Geometry: final body of the model. Coordinates: model frame, mm. A direction names the side the tool comes from. Round coordinates to 2 decimals unless told otherwise and drop trailing zeros. Write each loop counter-clockwise with the first axis right and the second up, starting at its lowest first coordinate (ties: lowest second). Pieces come first, ordered by that corner, then holes.
from build123d import *

# Parameters (mm, degrees)
SKETCH_R     = 3.65
PAD_DEPTH    = 31
SKETCH001_R  = 3.15
PAD001_DEPTH = 5
FILLET_R     = 1


with BuildPart() as part:
    # Sketch → Pad (new body)
    with BuildSketch(Plane.XY):
        Circle(SKETCH_R)
    extrude(amount=PAD_DEPTH)

    # Sketch001 (on Face3 of Pad) → Pad001 (join)
    with BuildSketch(Plane.XY.offset(31)):
        Circle(SKETCH001_R)
    extrude(amount=PAD001_DEPTH)

    # Fillet
    fillet_edges = [part.edges().sort_by_distance(p)[0] for p in [
        (-3.15, 0, 36),
    ]]
    fillet(fillet_edges, radius=FILLET_R)


solid = part.part
1) Section C-C on z = 9. Output: boundary loops of the cut face in (x, y).
2) Section A-A on x = 0. Output: boundary loops of the cut face in (y, z).
3) First-contact query: P1, Ø3, axis at x = -2.5, z = 23.5, coming from the -Y side; P2, Ø2, axis at x = 3, z = 31, coming from the -Y side. Flat tips, straight axial feed; report the tip coordinate or a pass-through.
4) Reachability of faces 3 (the cylindrical face through (-2.5, -1.917, 32.972)), 4 (the flat face through (0, 0, 36)) from +Z, -Z, +X, -X, +Y, -Y: full face, straight path, thin tool, end or side. Return the list, or none.
5) Draft query along X for faces 1 (the flat face through (0, 0, 0)), 2 (the cylindrical face through (3.48, 1.1, 15.28)). Return one class per face: pulls with the +X half, pulls with the -X half, needs draft (parallel to the pull), parting line crosses it, or undercut.
6) Line query: probe 1 along Z at (x, y) = (-1.75, -3); probe 2 along Z at (x, y) = (-1, -2); probe 3 along Y at (x, z) = (-2.25, 2). Output: solid intervals per line, ascending.
Filled in:
1. outline: circle Ø7.3 at (0, 0)
2. outline: (-3.65, 0) - (3.65, 0) - (3.65, 31) - (3.15, 31) - (3.15, 35) arc R1 ccw to (2.15, 36) - (-2.15, 36) arc R1 ccw to (-3.15, 35) - (-3.15, 31) - (-3.65, 31) - close
3. P1: stops at y = -3.51
3. P2: stops at y = -3.05
4. face 3: +Z
4. face 4: +Z, +X, -X, +Y, -Y
5. face 1: needs draft
5. face 2: parting line crosses it
6. probe 1: z = 0 to 31
6. probe 2: z = 0 to 36
6. probe 3: y = -2.87 to 2.87
